The model under review builds one solid part; all positions refer to its coordinate system, in mm. A direction names the side the tool comes from. Coordinates: 2 decimals unless noted, no trailing zeros. Order: outer loops, then holes, each group sorted by start corner. A loop starts at its lowest first (then second) coordinate and runs counter-clockwise, first axis right, second up. Notation, with made-up numbers: (76.25, 54) -> (83.25, 54) arc R27 ccw to (83.25, 88) -> close; hole circle Ø3 at (73.5, 20.5). An arc over 180 degrees is marked (long way). Use one line per item in the form item = value. Start each with the question number.
(1) Take a section at A-A (y = 107). State the section outline as (x, z) points.
(2) Wall thickness on line 1 along Z through (x, y) = (5, 78); line 2 along Z through (x, y) = (5, 23); line 3 along Y through (x, z) = (-32, -20): over which ranges is each line inside the solid? List them lowest first.
(3) Insertion check: pin 1 Ø4 at (y, z) = (29, 21.5) entering from +X; pin 2 Ø11.5 at (y, z) = (63, 28) entering from -X; pin 3 Ø2 at (y, z) = (69.5, 7.5) entering from -X. Each pin has a flat end and moves straight along its axis. Give the tip position at first contact, or say it passes through.
(4) Mouldability with a two-part tool opening along X and no side actions: class faces 1 (the flat face through (-22, 40.6, 0)), 2 (the cylindrical face through (-33.459, 141.944, -22.125)), 3 (the flat face through (-5, 69, -29)), 4 (the cylindrical face through (0.122, 120.605, -21.965)) as +X half, -X half, draft (parallel to the pull), parting line (faces both ways), or undercut.
(5) Take a section at B-B (z = 7.5). State how many separate pieces and enclosed holes the cut face has, then the cut area to 3 significant figures.
(6) For faces 5 (the flat face through (28, 25, -13)), 6 (the cylindrical face through (-42.25, 141.94, 0.31)), 7 (the flat face through (-23, 0, 0)), 8 (the flat face through (23.1, 138, 26.5)), 9 (the flat face through (-5, 69, 29)), list the 3-axis set-ups (+Z, -Z, +X, -X, +Y, -Y) from which the entire face can be reached by the end or side of a thin tool; tool diameter is ignored.
(7) Take a section at D-D (y = 62). State the section outline as (x, z) points, then the cut area to 3 significant figures.
```python
from build123d import *

# Parameters (mm, degrees)
CROQUIS1_R                = 35
SALIENTE_EXTRUIR1_DEPTH   = 138
CROQUIS2_R                = 45
SALIENTE_EXTRUIR2_DEPTH   = 8
CORTAR_EXTRUIR1_DEPTH     = 83.5
CORTAR_EXTRUIR2_DEPTH     = 167
TALADRO_ROSCADO_M41_D     = 3.3
TALADRO_ROSCADO_M41_DEPTH = 18
TALADRO_ROSCADO_M41_TIP   = 0.991420021


with BuildPart() as part:
    # Croquis1 → Saliente-Extruir1 (new body)
    with BuildSketch(Plane(origin=(0, 0, 0), x_dir=(1, 0, 0), z_dir=(0, 1, 0))):
        Circle(CROQUIS1_R)
    extrude(amount=SALIENTE_EXTRUIR1_DEPTH)

    # Croquis2 → Saliente-Extruir2 (add)
    with BuildSketch(Plane(origin=(0, 138, 0), x_dir=(1, 0, 0), z_dir=(0, 1, 0))):
        Circle(CROQUIS2_R)
    extrude(amount=SALIENTE_EXTRUIR2_DEPTH)

    # Croquis3 → Cortar-Revolución1 (revolve, cut)
    with BuildSketch(Plane.XY):
        Polygon((5, 0), (32.5, 0), (32.5, 22), (33.5, 22), (33.5, 25), (31, 25), (31, 113), (27.5, 113), (27.5, 128), (5, 141), align=None)
    revolve(axis=Axis((5, 141, 0), (0, -1, 0)), mode=Mode.SUBTRACT)

    # Croquis4 → Cortar-Extruir1 (cut, symmetric)
    with BuildSketch(Plane.XY):
        with BuildLine():
            Line((-35, 32.5), (-25.1, 40.6))
            Line((-25.1, 40.6), (-7, 40.6))
            ThreePointArc((-7, 40.6), (-5.585786438, 41.185786438), (-5, 42.6))
            Line((-5, 42.6), (-5, 95.2))
            ThreePointArc((-5, 95.2), (-5.585786438, 96.614213562), (-7, 97.2))
            Line((-7, 97.2), (-25.1, 97.2))
            Line((-25.1, 97.2), (-35, 105.3))
            Line((-35, 105.3), (-45, 105.3))
            Line((-45, 105.3), (-45, 32.5))
            Line((-45, 32.5), (-35, 32.5))
        make_face()
    extrude(amount=CORTAR_EXTRUIR1_DEPTH, both=True, mode=Mode.SUBTRACT)

    # Croquis5 → Cortar-Extruir2 (cut)
    with BuildSketch(Plane.XZ.offset(-138)):
        with BuildLine():
            ThreePointArc((-21.290820143, -36.493334702), (0, -42.25), (21.290820143, -36.493334702))
            ThreePointArc((21.290820143, -36.493334702), (22.10042151, -33.416072018), (19.023158826, -32.606470651))
            ThreePointArc((19.023158826, -32.606470651), (0, -37.75), (-19.023158826, -32.606470651))
            ThreePointArc((-19.023158826, -32.606470651), (-22.10042151, -33.416072018), (-21.290820143, -36.493334702))
        make_face()
        with BuildLine():
            ThreePointArc((36.493334702, -21.290820143), (42.25, 0), (36.493334702, 21.290820143))
            ThreePointArc((36.493334702, 21.290820143), (33.416072018, 22.10042151), (32.606470651, 19.023158826))
            ThreePointArc((32.606470651, 19.023158826), (37.75, 0), (32.606470651, -19.023158826))
            ThreePointArc((32.606470651, -19.023158826), (33.416072018, -22.10042151), (36.493334702, -21.290820143))
        make_face()
        with BuildLine():
            ThreePointArc((21.290820143, 36.493334702), (0, 42.25), (-21.290820143, 36.493334702))
            ThreePointArc((-21.290820143, 36.493334702), (-22.10042151, 33.416072018), (-19.023158826, 32.606470651))
            ThreePointArc((-19.023158826, 32.606470651), (0, 37.75), (19.023158826, 32.606470651))
            ThreePointArc((19.023158826, 32.606470651), (22.10042151, 33.416072018), (21.290820143, 36.493334702))
        make_face()
        with BuildLine():
            ThreePointArc((-36.493334702, 21.290820143), (-42.25, 0), (-36.493334702, -21.290820143))
            ThreePointArc((-36.493334702, -21.290820143), (-33.416072018, -22.10042151), (-32.606470651, -19.023158826))
            ThreePointArc((-32.606470651, -19.023158826), (-37.75, 0), (-32.606470651, 19.023158826))
            ThreePointArc((-32.606470651, 19.023158826), (-33.416072018, 22.10042151), (-36.493334702, 21.290820143))
        make_face()
    extrude(amount=-CORTAR_EXTRUIR2_DEPTH, mode=Mode.SUBTRACT)

    # Taladro roscado M41
    with Locations(Plane.XZ):
        with Locations((-30, 0)):
            Hole(TALADRO_ROSCADO_M41_D / 2, depth=TALADRO_ROSCADO_M41_DEPTH)
            with Locations((0, 0, -(TALADRO_ROSCADO_M41_DEPTH + TALADRO_ROSCADO_M41_TIP / 2))):  # 118° drill point
                Cone(0, TALADRO_ROSCADO_M41_D / 2, TALADRO_ROSCADO_M41_TIP, mode=Mode.SUBTRACT)


solid = part.part
```
Findings:
q1.outline = circle Ø70 at (0, 0); hole circle Ø52 at (5, 0)
q2.line_1 = -34.64 to -26, 26 to 34.64
q2.line_2 = -34.64 to -28.5, 28.5 to 34.64
q2.line_3 = 138 to 146
q3.pin_1 = 29.06
q3.pin_2 = -5
q3.pin_3 = 29.57
q4.face_1 = draft
q4.face_2 = undercut
q4.face_3 = -X half
q4.face_4 = undercut
q5.separate_pieces = 4
q5.enclosed_holes = 0
q5.area = 2,630 mm²
q6.face_5 = none
q6.face_6 = +Y, -Y
q6.face_7 = +Z, -Z, +X, -X, -Y
q6.face_8 = -Y
q6.face_9 = +Z, -Z, -X
q7.outline = (-5, -34.64) arc R35 ccw (long way) to (-5, 34.64) -> (-5, 24) arc R26 cw (long way) to (-5, -24) -> close
q7.area = 704 mm²
